The drawing under review shows one solid part. Ordinate dimensions are in mm from its lowest x, y, z. A direction names the side the tool comes from. Give positions to 0.01 mm unless a question says otherwise; leave off trailing zeros. Order: outer loops, then holes, each group sorted by start corner. A loop starts at its lowest first (then second) coordinate and runs counter-clockwise, first axis right, second up. Notation, with made-up numbers: M 38.25,24.25 L 92.25,24.25 A16 cw 92.25,50.25 Z; hole C -17.75,12 d2. An arc over 180 degrees is marked long. Put each result on its own line as item: value. Start each with the question number.
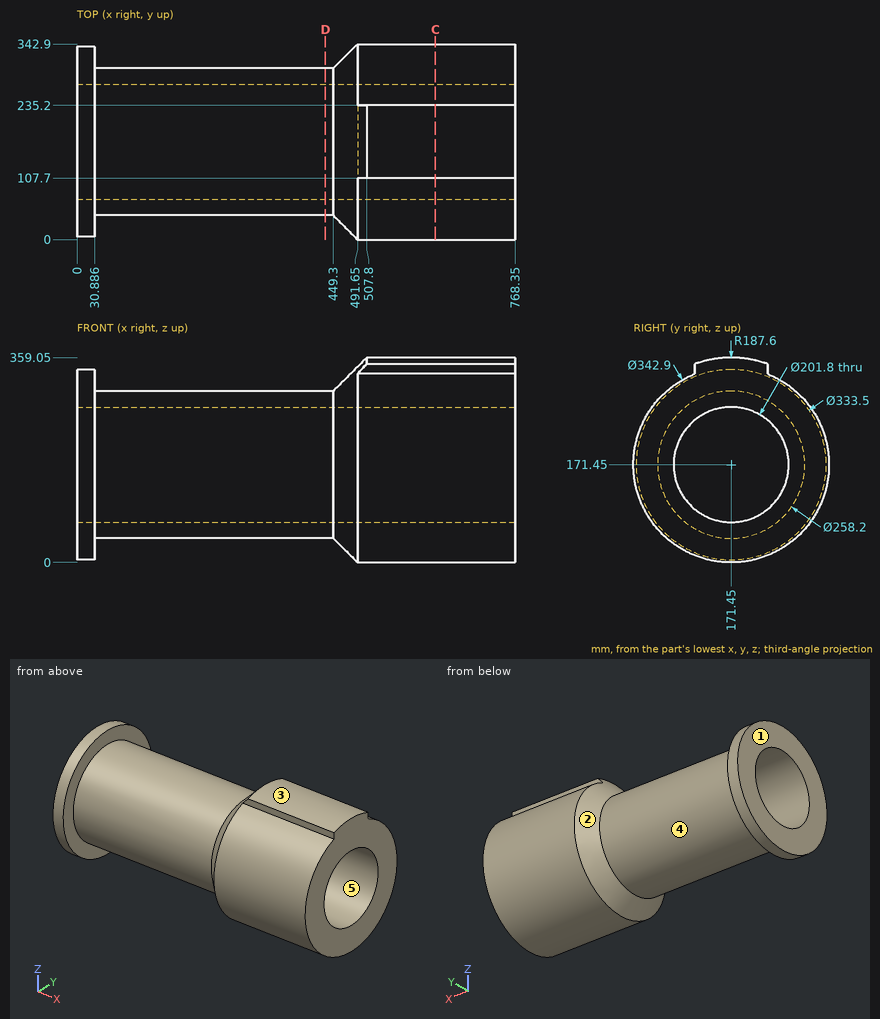
1. Consider section D-D on x = 435.5. Give the boundary of the cut face in (y, z), then the cut area to 3 significant figures.
2. Machinability: for the marked faces 1 and 2, which of the approach directions +Z, -Z, +X, -X, +Y, -Y give a long, thin tool a straight path to every point of the face, cutting with its end or side? Answer none if there is none.
3. Insertion check: pin 1 (2 mm diameter, centred on x = 685.5, y = 266, fed in from +Z); pin 2 (12 mm diameter, centred on x = 456.5, z = 247, fed in from +Y); pin 3 (1 mm diameter, centred on x = 84.5, y = 53.5, fed in from +Z) (1 decimal). Each pin has a flat end and moves straight along its axis. Give the tip position at first contact, or say it passes through.
4. The part is to be moulded in two halves that separate along Z. For the marked faces 3, 4 and 5, say which applies: +Z half, -Z half, draft (parallel to the pull), parting line (faces both ways), or undercut.
5. To check wall thickness, follow probe 1 along Y at (x, z) = (207, 171); probe 2 along Y at (x, z) = (535, 171). State the ranges of each line that lie inside material, in increasing order.
6. Consider section C-C on x = 628. Give the boundary of the cut face in (y, z).
Returned:
1. outline: C 171.45,171.45 d258.2; hole C 171.45,171.45 d201.8
1. area: 20,400 mm2
2. face 1: +Z, -Z, -X, +Y, -Y
2. face 2: none
3. pin 1: stops at z = 315.13
3. pin 2: stops at y = 292.94
3. pin 3: stops at z = 225
4. face 3: +Z half
4. face 4: parting line
4. face 5: undercut
5. probe 1: y = 42.35 to 70.55, 272.35 to 300.55
5. probe 2: y = 0 to 70.55, 272.35 to 342.9
6. outline: M 107.7,330.61 A171.45 ccw long 235.2,330.61 L 235.2,347.89 A187.6 ccw 107.7,347.89 Z; hole C 171.45,171.45 d201.8
